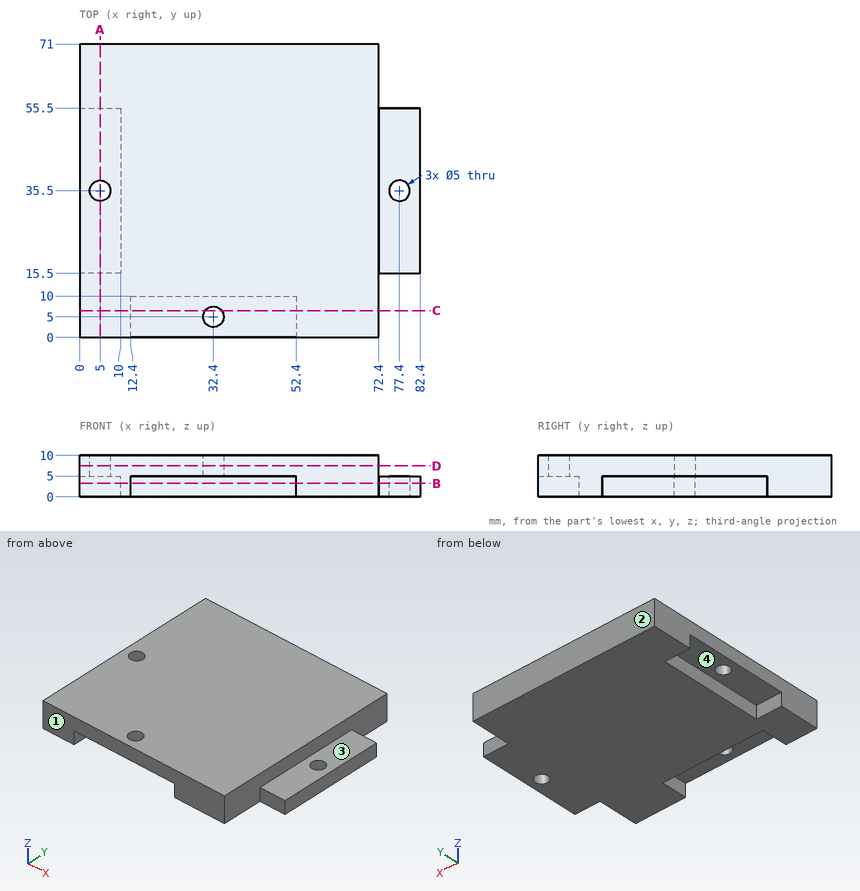
Design review of the part shown in the three views and the two pictorial views. Dimensions are in mm from the part's minimum x, y and z. Round coordinates to 2 decimals unless told otherwise and drop trailing zeros. Loops run counter-clockwise (first coordinate to the right, second up) from the corner with the lowest first, then second, coordinate; pieces in that order, holes last. Notation, with made-up numbers: (-3.75, -21.5) - (43.25, -21.5) arc R31 ccw to (43.25, 5.5) - close; hole circle Ø11 at (84.5, 13). An arc over 180 degrees is marked (long way). One line per item, written item: value. Start each with the question number.
Item 1: Take a section at C-C (y = 6.5). Give the boundary of the cut face in (x, z).
Item 2: Clearance check with flat-ended pins moving along their axes: pin 1 Ø1.5 at (x, z) = (2.5, 2) entering from -Y; pin 2 Ø4 at (x, y) = (5, 35.5) entering from -Z; pin 3 Ø3 at (x, y) = (39, 5) entering from -Z; pin 4 Ø1.5 at (y, z) = (35, 2.5) entering from -X. State where each tip first meets the part, or that it passes through.
Item 3: The part is to be moulded in two halves that separate along Y. For the marked faces 1, 2, 3 and 4, say which applies: +Y half, -Y half, draft (parallel to the pull), parting line (faces both ways), or undercut.
Item 4: Take a section at B-B (z = 3.25). Give the boundary of the cut face in (x, y), plus the area to 3 significant figures.
Item 5: For L1, parallel to X at y = 6, z = 2.25; L2, parallel to Y at x = 5, z = 6.75; L3, parallel to Y at x = 77.4, z = 4, list the stretches that pass through material, from the lowest coordinate up.
Item 6: Take a section at D-D (z = 7.5). Give the boundary of the cut face in (x, y), plus the area to 3 significant figures.
Item 7: Take a section at A-A (x = 5). Give the boundary of the cut face in (y, z).
Answer below:
1. outline: (0, 0) - (12.4, 0) - (12.4, 5) - (30.4, 5) - (30.4, 10) - (0, 10) - close; (34.4, 5) - (52.4, 5) - (52.4, 0) - (72.4, 0) - (72.4, 10) - (34.4, 10) - close
2. pin 1: stops at y = 0
2. pin 2: passes through
2. pin 3: stops at z = 5
2. pin 4: stops at x = 10
3. face 1: -Y half
3. face 2: +Y half
3. face 3: draft
3. face 4: undercut
4. outline: (0, 0) - (12.4, 0) - (12.4, 10) - (52.4, 10) - (52.4, 0) - (72.4, 0) - (72.4, 15.5) - (82.4, 15.5) - (82.4, 55.5) - (72.4, 55.5) - (72.4, 71) - (0, 71) - (0, 55.5) - (10, 55.5) - (10, 15.5) - (0, 15.5) - close; hole circle Ø5 at (77.4, 35.5)
4. area: 4,720 mm2
5. L1: x = 0 to 12.4, 52.4 to 72.4
5. L2: y = 0 to 33, 38 to 71
5. L3: y = 15.5 to 33, 38 to 55.5
6. outline: (0, 0) - (72.4, 0) - (72.4, 71) - (0, 71) - close; hole circle Ø5 at (5, 35.5); hole circle Ø5 at (32.4, 5)
6. area: 5,100 mm2
7. outline: (0, 0) - (15.5, 0) - (15.5, 5) - (33, 5) - (33, 10) - (0, 10) - close; (38, 5) - (55.5, 5) - (55.5, 0) - (71, 0) - (71, 10) - (38, 10) - close
